```python
from build123d import *

# Parameters (mm, degrees)
SKETCH_R          = 10
PAD_DEPTH         = 50
PAD_DEPTH_BACK    = 50
SKETCH001_R       = 6
PAD001_DEPTH      = 90
POCKET_DEPTH      = 80
SKETCH003_R       = 4
PAD002_DEPTH      = 1
PAD002_DEPTH_BACK = 90


with BuildPart() as part:
    # Sketch → Pad (new body, two sides)
    with BuildSketch(Plane.XY) as pad_sk:
        Circle(SKETCH_R)
    extrude(amount=PAD_DEPTH)
    extrude(pad_sk.sketch, amount=-PAD_DEPTH_BACK)

    # Sketch001 → Pad001 (join)
    with BuildSketch(Plane.XY):
        Circle(SKETCH001_R)
    extrude(amount=PAD001_DEPTH)

    # Sketch002 (on Face7 of Pad001) → Pocket (cut)
    with BuildSketch(Plane.XY.offset(70)):
        with BuildLine():
            ThreePointArc((2.549937, -1.580449), (-1.766635, 2.424665), (0.722998, -2.911576))
            Line((0.722998, -2.911576), (2.549937, -1.580449))
        make_face()
    extrude(amount=POCKET_DEPTH, mode=Mode.SUBTRACT)

    # Sketch003 → Pad002 (join, two sides)
    with BuildSketch(Plane.XY) as pad002_sk:
        Circle(SKETCH003_R)
    extrude(amount=PAD002_DEPTH)
    extrude(pad002_sk.sketch, amount=-PAD002_DEPTH_BACK)


solid = part.part
```
Model file for the job. Use its own axes, mm. A direction names the side the tool comes from. Give positions to 0.01 mm unless a question says otherwise; leave off trailing zeros. Write each loop counter-clockwise with the first axis right and the second up, starting at its lowest first coordinate (ties: lowest second). Pieces come first, ordered by that corner, then holes. Notation, with made-up numbers: (-3.5, 9) -> (51.5, 9) arc R26 ccw to (51.5, 27) -> close; hole circle Ø7 at (-29.5, -38). An arc over 180 degrees is marked (long way). Use CSV: the item, a comma, the result in double quotes. Start each with the question number.
1) Pin check, flat tips, straight feed: P1, Ø1, axis at y = -5.5, z = 67.5, coming from the -X side; P2, Ø1.5, axis at x = 7, z = -28.5, coming from the -Y side. Stop position of each tip, or through.
2) Cut at B-B on z = 25. List the corners of the cut face in (x, y), plus the area to 3 significant figures.
3) Tool access for faces 4 (the cylindrical face through (-2.17, -9.76, 0.7)), 5 (the flat face through (-0.1, -4.3, -50)), 6 (the cylindrical face through (-6, 0, 70)): list every direction of +Z, -Z, +X, -X, +Y, -Y with a clear straight run to the whole face (end or side of a thin tool).
4) Cut at C-C on x = 8. List the corners of the cut face in (y, z), plus the area to 3 significant figures.
5) Two-plate mould, pull along Y, no slides. Class faces 1 (the flat face through (0, 0, -90)), 2 (the cylindrical face through (-0.867, -3.905, -69.72)), 3 (the cylindrical face through (-1.67, 2.49, 79.86)): released by +Y, released by -Y, zero draft, split by the parting line, or undercut.
6) Drill centre lines: L1, parallel to Y at x = 0, z = 76.75; L2, parallel to Z at x = -3, y = -5.25. Where is each one in solid material? Low to high.
7) Cut at D-D on z = -53.5. List the corners of the cut face in (x, y).
8) Cut at A-A on y = 0. List the corners of the cut face in (x, z), plus the area to 3 significant figures.
Final values:
1,P1,"stops at x = -3.32"
1,P2,"stops at y = -7.81"
2,outline,"circle Ø20 at (0, 0)"
2,area,"314 mm2"
3,face 4,"+Z, -Z"
3,face 5,"-Z"
3,face 6,"+Z"
4,outline,"(-6, -50) -> (6, -50) -> (6, 50) -> (-6, 50) -> close"
4,area,"1,200 mm2"
5,face 1,"zero draft"
5,face 2,"split by the parting line"
5,face 3,"undercut"
6,L1,"y = -6 to -3, 3 to 6"
6,L2,"z = -50 to 50"
7,outline,"circle Ø8 at (0, 0)"
8,outline,"(-10, -50) -> (-4, -50) -> (-4, -90) -> (4, -90) -> (4, -50) -> (10, -50) -> (10, 50) -> (6, 50) -> (6, 90) -> (3, 90) -> (3, 70) -> (-3, 70) -> (-3, 90) -> (-6, 90) -> (-6, 50) -> (-10, 50) -> close"
8,area,"2,680 mm2"
